```python
from build123d import *

# Parameters (mm, degrees)
SKETCH1_R           = 6.35
SKETCH1_R_2         = 2.54
BOSS_EXTRUDE1_DEPTH = 1.5875


with BuildPart() as part:
    # Sketch1 → Boss-Extrude1 (new body)
    with BuildSketch(Plane.XY):
        with BuildLine():
            Line((0, 0), (139.7, 0))
            ThreePointArc((139.7, 0), (165.1, 25.4), (139.7, 50.8))
            Line((139.7, 50.8), (0, 50.8))
            Line((0, 50.8), (0, 0))
        make_face()
        with Locations((146.05, 25.4)):
            Circle(SKETCH1_R, mode=Mode.SUBTRACT)
        with Locations((25.4, 25.4)):
            Circle(SKETCH1_R_2, mode=Mode.SUBTRACT)
        with Locations((76.2, 25.4)):
            Circle(SKETCH1_R_2, mode=Mode.SUBTRACT)
        with Locations((127, 25.4)):
            Circle(SKETCH1_R_2, mode=Mode.SUBTRACT)
    extrude(amount=BOSS_EXTRUDE1_DEPTH)


solid = part.part
```
Geometry: final body of the model. Coordinates: model frame, mm. Round coordinates to 2 decimals unless told otherwise and drop trailing zeros. Write each loop counter-clockwise with the first axis right and the second up, starting at its lowest first coordinate (ties: lowest second). Pieces come first, ordered by that corner, then holes. Notation, with made-up numbers: (69, 73.25) -> (99, 73.25) arc R10 cw to (99, 92.25) -> close; hole circle Ø10 at (-7, -26). An arc over 180 degrees is marked (long way). Return JSON: item names as keys, results as strings.
Q1. Ray query, line 1 (Y direction, x = 76.5, z = 1.3); line 2 (Y direction, x = 128.5, z = 1); line 3 (X direction, y = 4, z = 1.5). Return the intervals inside material, ascending.
From the geometry:
{"line 1": "0 to 22.88, 27.92 to 50.8", "line 2": "0 to 23.35, 27.45 to 50.8", "line 3": "0 to 153.38"}
Q2. First-contact query: pin 1 Ø4.5 at (x, y) = (127, 25.4) entering from -Z. Flat tip, straight axial feed; report the tip coordinate or a pass-through.
From the geometry:
{"pin 1": "through"}
Q3. Mould query, pull axis X, two halves, no side actions, for faces 1 (the cylindrical face through (141.01, 21.54, 0.78)), 2 (the cylindrical face through (74.33, 27.12, 0.78)), 3 (the flat face through (81, 26, 0)), 4 (the cylindrical face through (165.094, 24.841, 0.783)). Classes: +X half, -X half, draft (parallel to the pull), parting line (faces both ways), or undercut.
From the geometry:
{"face 1": "undercut", "face 2": "undercut", "face 3": "draft", "face 4": "+X half"}
Q4. Section D-D on y = 5.5. Return the cut outline in (x, z), and give its area (3 significant figures).
From the geometry:
{"outline": "(0, 0) -> (155.48, 0) -> (155.48, 1.59) -> (0, 1.59) -> close", "area": "247 mm2"}
Q5. Section C-C on x = 127.5. Return the cut outline in (y, z).
From the geometry:
{"outline": "(0, 0) -> (22.91, 0) -> (22.91, 1.59) -> (0, 1.59) -> close; (27.89, 0) -> (50.8, 0) -> (50.8, 1.59) -> (27.89, 1.59) -> close"}
Q6. Section B-B on x = 25.4. Return the cut outline in (y, z).
From the geometry:
{"outline": "(0, 0) -> (22.86, 0) -> (22.86, 1.59) -> (0, 1.59) -> close; (27.94, 0) -> (50.8, 0) -> (50.8, 1.59) -> (27.94, 1.59) -> close"}
Q7. Section A-A on y = 25.4. Return the cut outline in (x, z), and give its area (3 significant figures).
From the geometry:
{"outline": "(0, 0) -> (22.86, 0) -> (22.86, 1.59) -> (0, 1.59) -> close; (27.94, 0) -> (73.66, 0) -> (73.66, 1.59) -> (27.94, 1.59) -> close; (78.74, 0) -> (124.46, 0) -> (124.46, 1.59) -> (78.74, 1.59) -> close; (129.54, 0) -> (139.7, 0) -> (139.7, 1.59) -> (129.54, 1.59) -> close; (152.4, 0) -> (165.1, 0) -> (165.1, 1.59) -> (152.4, 1.59) -> close", "area": "218 mm2"}
